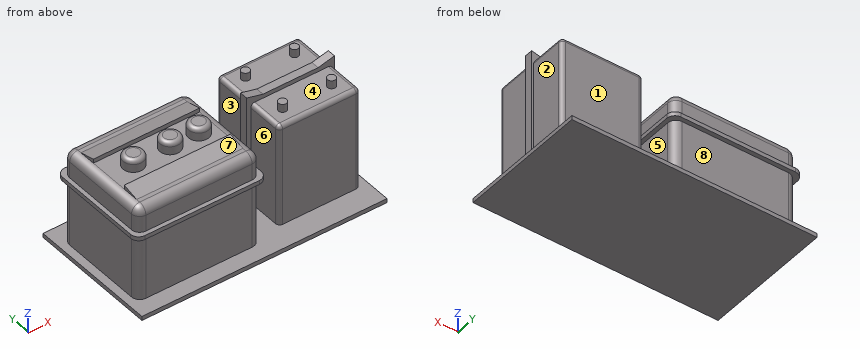
from build123d import *

# Parameters (mm, degrees)
F1_W      = 30
F1_H      = 24
F2_DEPTH  = 24
F3_R      = 2
F4_W      = 32
F4_H      = 1
F5_DEPTH  = 13
F6_R      = 2
F7_R      = 2.5
F8_DEPTH  = 3
F9_R      = 1
F11_DEPTH = 26
F13_W     = 20
F13_H     = 20
F14_DEPTH = 26
F15_R     = 1
F16_R     = 1
F17_DEPTH = 2
F19_DEPTH = 1
F20_W     = 60
F20_H     = 32
F21_DEPTH = 1


with BuildPart() as f2:
    # F1 (on Top) → F2 (new body)
    with BuildSketch(Plane.XY):
        with Locations((-15, 0)):
            Rectangle(F1_W, F1_H)
    extrude(amount=F2_DEPTH)

    # F3
    f3_edges = [f2.edges().sort_by_distance(p)[0] for p in [
        (-30, 12, 12),
        (0, 12, 12),
        (-30, -12, 12),
        (0, -12, 12),
        (-15, 12, 24),
        (-30, 0, 24),
        (-15, -12, 24),
        (0, 0, 24),
    ]]
    fillet(f3_edges, radius=F3_R)

    # F4 (on Front) → F5 (join, symmetric)
    with BuildSketch(Plane.XZ):
        with Locations((-15, 17.5)):
            Rectangle(F4_W, F4_H)
    extrude(amount=F5_DEPTH, both=True)

    # F6
    f6_edges = [f2.edges().sort_by_distance(p)[0] for p in [
        (-31, 13, 17.5),
        (-31, -13, 17.5),
        (1, 13, 17.5),
        (1, -13, 17.5),
    ]]
    fillet(f6_edges, radius=F6_R)

    # F7 (on face) → F8 (join)
    with BuildSketch(Plane.XY.offset(24)):
        with Locations((-22, 0)):
            Circle(F7_R)
        with Locations((-13, 0)):
            Circle(F7_R)
        with Locations((-6, 0)):
            Circle(F7_R)
    extrude(amount=F8_DEPTH)

    # F9
    f9_edges = [f2.edges().sort_by_distance(p)[0] for p in [
        (-24.5, 0, 27),
        (-15.5, 0, 27),
        (-8.5, 0, 27),
    ]]
    fillet(f9_edges, radius=F9_R)

    # F10 (on offset) → F11 (join)
    with BuildSketch(Plane.YZ.offset(-2)):
        Polygon((-9, 24), (-5, 24), (-5, 25), align=None)
    extrude(amount=-F11_DEPTH)

    # F12: F2 across plane


with BuildPart() as f2_1:
    add(f2.part)
    add(f2.part.mirror(Plane.XZ))



with BuildPart() as f14:
    # F13 (on Top) → F14 (new body)
    with BuildSketch(Plane.XY):
        with Locations((16, 0)):
            Rectangle(F13_W, F13_H)
    extrude(amount=F14_DEPTH)

    # F15
    f15_edges = [f14.edges().sort_by_distance(p)[0] for p in [
        (26, 10, 13),
        (16, 10, 26),
        (6, 0, 26),
        (16, -10, 26),
        (26, 0, 26),
        (26, -10, 13),
        (6, 10, 13),
        (6, -10, 13),
    ]]
    fillet(f15_edges, radius=F15_R)

    # F16 (on face) → F17 (join)
    with BuildSketch(Plane.XY.offset(26)):
        with Locations((10, 6)):
            Circle(F16_R)
        with Locations((22, 6)):
            Circle(F16_R)
        with Locations((10, -6)):
            Circle(F16_R)
        with Locations((22, -6)):
            Circle(F16_R)
    extrude(amount=F17_DEPTH)

    # F18 (on Front) → F19 (join, symmetric)
    with BuildSketch(Plane.XZ):
        Polygon((5, 28), (5, 0), (26.5, 0), (26.5, 28), (22.5, 27), (9, 27), align=None)
    extrude(amount=F19_DEPTH, both=True)


with BuildPart() as f2_2:
    add(f2_1.part)

    add(f14.part)  # F21 merges F14
    # F20 (on Top) → F21 (join)
    with BuildSketch(Plane.XY):
        with Locations((-2, 0)):
            Rectangle(F20_W, F20_H)
    extrude(amount=F21_DEPTH)


solid = f2_2.part
The listing builds one solid part. Answer for the finished solid, in the listing's coordinates (mm). Face numbers are marked on the shaded views. A direction names the side the tool comes from. Give positions to 0.01 mm unless a question says otherwise; leave off trailing zeros. Loops run counter-clockwise (first coordinate to the right, second up) from the corner with the lowest first, then second, coordinate; pieces in that order, holes last.
Item 1: Each of these flat-tipped pins is pushed along its axis until it touches: pin 1 Ø2 at (x, y) = (-10.5, -1) entering from +Z; pin 2 Ø0.5 at (y, z) = (-7, 24.5) entering from -X; pin 3 Ø1.1 at (x, y) = (-21, -9.5) entering from +Z. Where does it stop, or does it pass through?
Derived:
pin 1: stops at z = 26.98
pin 2: stops at x = -28
pin 3: stops at z = 24.01
Item 2: A tool of negligible diameter and unlimited length cuts with its end or side. For the marked faces 5, 6, 7 and 8, from which of +Z, -Z, +X, -X, +Y, -Y can it reach the whole face along a straight path? Write none if from no direction.
Derived:
face 5: +Y, -Y
face 6: +Z, -Y
face 7: +Z, -X, -Y
face 8: +X, -X, +Y
Item 3: A cutting plane is placed at A-A (z = 19.5). Give the vertices of the cut face in (x, y).
Derived:
outline: (-30, -10) arc R2 ccw to (-28, -12) - (-2, -12) arc R2 ccw to (0, -10) - (0, 10) arc R2 ccw to (-2, 12) - (-28, 12) arc R2 ccw to (-30, 10) - close; (5, -1) - (6, -1) - (6, -9) arc R1 ccw to (7, -10) - (25, -10) arc R1 ccw to (26, -9) - (26, -1) - (26.5, -1) - (26.5, 1) - (26, 1) - (26, 9) arc R1 ccw to (25, 10) - (7, 10) arc R1 ccw to (6, 9) - (6, 1) - (5, 1) - close
Item 4: A cutting plane is placed at D-D (x = 24). Give the vertices of the cut face in (y, z) (3 decimals).
Derived:
outline: (-16, 0) - (16, 0) - (16, 1) - (10, 1) - (10, 25) arc R1 ccw to (9, 26) - (1, 26) - (1, 27.375) - (-1, 27.375) - (-1, 26) - (-9, 26) arc R1 ccw to (-10, 25) - (-10, 1) - (-16, 1) - close
Item 5: Determine the mould class of the marked faces 1, 2, 3 and 4 for opening direction X: +X half, -X half, draft (parallel to the pull), parting line (faces both ways), or undercut.
Derived:
face 1: draft
face 2: +X half
face 3: undercut
face 4: undercut
Item 6: A cutting plane is placed at B-B (x = 10). Give the vertices of the cut face in (y, z), then the cut area to 3 significant figures.
Derived:
outline: (-16, 0) - (16, 0) - (16, 1) - (10, 1) - (10, 25) arc R1 ccw to (9, 26) - (7, 26) - (7, 28) - (5, 28) - (5, 26) - (1, 26) - (1, 27) - (-1, 27) - (-1, 26) - (-5, 26) - (-5, 28) - (-7, 28) - (-7, 26) - (-9, 26) arc R1 ccw to (-10, 25) - (-10, 1) - (-16, 1) - close
area: 542 mm2
Item 7: Find the intervals of material crossed by line 1 along X through (y, z) = (7, 17.5); line 2 along X through (y, z) = (-2, 13.25); line 3 along Y through (x, z) = (-16, 15.25), in increasing order.
Derived:
line 1: x = -31 to 1, 6 to 26
line 2: x = -30 to 0, 6 to 26
line 3: y = -12 to 12
